Input: part model. Units: mm. Frame: model coordinates. Coordinates: 2 decimals unless noted, no trailing zeros. Loops run counter-clockwise (first coordinate to the right, second up) from the corner with the lowest first, then second, coordinate; pieces in that order, holes last. Notation, with made-up numbers: (34, 69) -> (75, 69) arc R9 cw to (75, 79) -> close; hole circle Ø8 at (23, -25.75). An arc over 180 degrees is marked (long way). Answer as a JSON object with one key per item and string values.
from build123d import *

# Parameters (mm, degrees)
BOSS_EXTRUDE1_DEPTH = 6.35


with BuildPart() as part:
    # Sketch1 → Boss-Extrude1 (new body)
    with BuildSketch(Plane(origin=(0, 0, 0), x_dir=(1, 0, 0), z_dir=(0, 1, 0))):
        with BuildLine():
            Line((209.55, 0), (428.625, 0))
            ThreePointArc((428.625, 0), (437.605256121, 3.719743879), (441.325, 12.7))
            Line((441.325, 12.7), (441.325, 58.239487758))
            ThreePointArc((441.325, 58.239487758), (442.291729937, 63.099567349), (445.044743879, 67.219743879))
            Line((445.044743879, 67.219743879), (570.955256121, 193.130256121))
            ThreePointArc((570.955256121, 193.130256121), (575.075432651, 195.883270063), (579.935512242, 196.85))
            Line((579.935512242, 196.85), (625.475, 196.85))
            ThreePointArc((625.475, 196.85), (634.455256121, 200.569743879), (638.175, 209.55))
            Line((638.175, 209.55), (638.175, 358.775))
            Line((638.175, 358.775), (638.175, 460.375))
            Line((638.175, 460.375), (638.175, 530.225))
            ThreePointArc((638.175, 530.225), (634.455256121, 539.205256121), (625.475, 542.925))
            Line((625.475, 542.925), (579.935512242, 542.925))
            ThreePointArc((579.935512242, 542.925), (575.075432651, 543.891729937), (570.955256121, 546.644743879))
            Line((570.955256121, 546.644743879), (445.044743879, 672.555256121))
            ThreePointArc((445.044743879, 672.555256121), (442.291729937, 676.675432651), (441.325, 681.535512242))
            Line((441.325, 681.535512242), (441.325, 727.075))
            ThreePointArc((441.325, 727.075), (437.605256121, 736.055256121), (428.625, 739.775))
            Line((428.625, 739.775), (209.55, 739.775))
            ThreePointArc((209.55, 739.775), (200.569743879, 736.055256121), (196.85, 727.075))
            Line((196.85, 727.075), (196.85, 681.535512242))
            ThreePointArc((196.85, 681.535512242), (195.883270063, 676.675432651), (193.130256121, 672.555256121))
            Line((193.130256121, 672.555256121), (67.219743879, 546.644743879))
            ThreePointArc((67.219743879, 546.644743879), (63.099567349, 543.891729937), (58.239487758, 542.925))
            Line((58.239487758, 542.925), (12.7, 542.925))
            ThreePointArc((12.7, 542.925), (3.719743879, 539.205256121), (0, 530.225))
            Line((0, 530.225), (0, 209.55))
            ThreePointArc((0, 209.55), (3.719743879, 200.569743879), (12.7, 196.85))
            Line((12.7, 196.85), (58.239487758, 196.85))
            ThreePointArc((58.239487758, 196.85), (63.099567349, 195.883270063), (67.219743879, 193.130256121))
            Line((67.219743879, 193.130256121), (193.130256121, 67.219743879))
            ThreePointArc((193.130256121, 67.219743879), (195.883270063, 63.099567349), (196.85, 58.239487758))
            Line((196.85, 58.239487758), (196.85, 12.7))
            ThreePointArc((196.85, 12.7), (200.569743879, 3.719743879), (209.55, 0))
        make_face()
        with BuildLine():
            Line((619.125, 460.375), (568.325, 460.375))
            ThreePointArc((568.325, 460.375), (563.834871939, 458.515128061), (561.975, 454.025))
            Line((561.975, 454.025), (561.975, 365.125))
            ThreePointArc((561.975, 365.125), (563.834871939, 360.634871939), (568.325, 358.775))
            Line((568.325, 358.775), (619.125, 358.775))
            ThreePointArc((619.125, 358.775), (623.615128061, 360.634871939), (625.475, 365.125))
            Line((625.475, 365.125), (625.475, 454.025))
            ThreePointArc((625.475, 454.025), (623.615128061, 458.515128061), (619.125, 460.375))
        make_face(mode=Mode.SUBTRACT)
        with BuildLine():
            Line((12.7, 454.025), (12.7, 365.125))
            ThreePointArc((12.7, 365.125), (14.559871939, 360.634871939), (19.05, 358.775))
            Line((19.05, 358.775), (69.85, 358.775))
            ThreePointArc((69.85, 358.775), (74.340128061, 360.634871939), (76.2, 365.125))
            Line((76.2, 365.125), (76.2, 454.025))
            ThreePointArc((76.2, 454.025), (74.340128061, 458.515128061), (69.85, 460.375))
            Line((69.85, 460.375), (19.05, 460.375))
            ThreePointArc((19.05, 460.375), (14.559871939, 458.515128061), (12.7, 454.025))
        make_face(mode=Mode.SUBTRACT)
    extrude(amount=BOSS_EXTRUDE1_DEPTH)


solid = part.part
1. Section query B-B (x = 507). Return loops of the section in (y, z) (3 decimals).
Reply:
{"outline": "(0, -610.6) -> (6.35, -610.6) -> (6.35, -129.175) -> (0, -129.175) -> close"}
2. Section query A-A (y = 3.5). Count the separate pieces of the cut face and the enclosed holes in it, plus the area to 3 significant figures.
Reply:
{"separate pieces": "1", "enclosed holes": "2", "area": "340,000 mm2"}
3. Line query: line 1 along X through (y, z) = (2, -373) (3 decimals); line 2 along Z through (x, y) = (590, 3.75) (3 decimals); line 3 along Z through (x, y) = (565, 6) (3 decimals). Output: solid intervals per line, ascending.
Reply:
{"line 1": "x = 0 to 12.7, 76.2 to 561.975, 625.475 to 638.175", "line 2": "z = -542.925 to -460.375, -358.775 to -196.85", "line 3": "z = -552.6 to -459.435, -359.715 to -187.175"}
4. Pin query (flat end, axial travel): P1, Ø3, axis at x = 584, y = 3.5, coming from the +Z side; P2, Ø4, axis at x = 437.5, z = -661, coming from the -Y side; P3, Ø1.9, axis at y = 3, z = -35.5, coming from the -X side; P4, Ø1.9, axis at x = 24, y = 2.5, coming from the -Z side (3 decimals). Return the tip coordinate at first contact, or that it passes through.
Reply:
{"P1": "stops at z = -196.85", "P2": "stops at y = 0", "P3": "stops at x = 196.85", "P4": "stops at z = -542.925"}
5. Section query C-C (z = -119). Return loops of the section in (x, y) (3 decimals), plus the area to 3 significant figures.
Reply:
{"outline": "(141.35, 0) -> (496.825, 0) -> (496.825, 6.35) -> (141.35, 6.35) -> close", "area": "2,260 mm2"}
